from build123d import *

# Parameters (mm, degrees)
F0_W     = 261.6643384099
F0_H     = 143.3737166226
F1_DEPTH = 5
F2_R     = 19.4105187662
F3_DEPTH = 2
F6_R     = 6.5980928428
F7_DEPTH = 96.0488122602


# Not quite as in the source:
# - a feature of the source that left no trace in its solid (it failed there, or was rolled back) is left out


with BuildPart() as f1:
    # F0 (on Top) → F1 (new body)
    with BuildSketch(Plane.XY):
        with Locations((-11.2871490419, -11.1323576421)):
            Rectangle(F0_W, F0_H)
    extrude(amount=F1_DEPTH)

    # F2 (on face) → F3 (cut)
    with BuildSketch(Plane.XY.offset(5)):
        with Locations((-101.0480299592, -26.7270803452)):
            Circle(F2_R)
    extrude(amount=-F3_DEPTH, mode=Mode.SUBTRACT)


with BuildPart() as f7:
    # F6 (on line) → F7 (new body, through all)
    with BuildSketch(Plane(origin=(41.3091172937, 0, 32.6350144213), x_dir=(0, 1, 0), z_dir=(0.7846743667, 0, 0.6199081692))):
        with Locations((0, 4.5975914841)):
            Circle(F6_R)
    extrude(amount=-F7_DEPTH)


with BuildPart() as f1_1:
    add(f1.part)

    # F8: cut F7
    add(f7.part, mode=Mode.SUBTRACT)


solid = f1_1.part
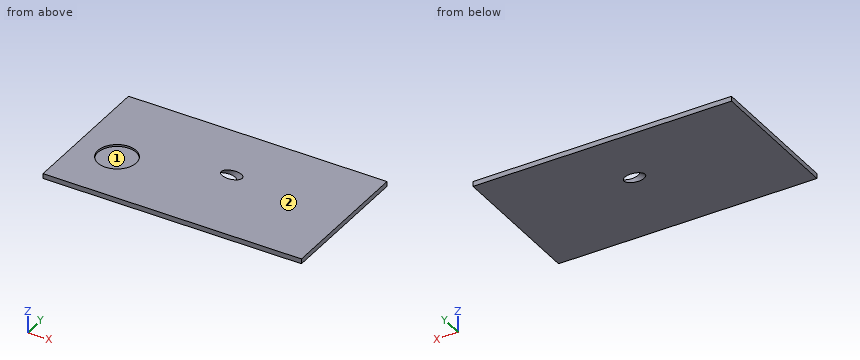
Verification items for the finished model (mm, model axes). Face numbers are marked on the shaded views. Give positions to 0.01 mm unless a question says otherwise; leave off trailing zeros. Loops run counter-clockwise (first coordinate to the right, second up) from the corner with the lowest first, then second, coordinate; pieces in that order, holes last. Notation, with made-up numbers: (-28, 20.25) - (-18, 20.25) arc R27 cw to (-18, 42.25) - close; hole circle Ø4 at (-27, -7). An arc over 180 degrees is marked (long way). Write item = value, one per line. Start each with the question number.
Q1. Cross-section at A-A, the plane y = 3. Enter the section's corners in (x, z).
Q2. Mould release check, pull along X, two halves, no side actions. Record for the marked faces 1 and 2: released by +X, released by -X, zero draft, split by the parting line, or undercut.
Q3. Thickness scan on line 1 (Y direction, x = -11, z = 1.1); line 2 (Y direction, x = -91, z = 3.65). Record the ranges inside material, lowest first.
Q4. Cross-section at B-B, the plane y = -32. Enter the section's corners in (x, z), and give its area (3 significant figures).
Q5. Cross-section at C-C, the plane z = 3.85. State how many separate pieces and enclosed holes the cut face has, and give its area (3 significant figures).
Answer key:
q1.outline = (-142.12, 0) - (-16.9, 0) - (-10.57, 5) - (-142.12, 5) - close; (2.06, 0) - (119.55, 0) - (119.55, 5) - (8.39, 5) - close
q2.face_1 = undercut
q2.face_2 = zero draft
q3.line_1 = -82.82 to -5.83, 5.83 to 60.55
q3.line_2 = -82.82 to -43.33, -10.12 to 60.55
q4.outline = (-142.12, 0) - (119.55, 0) - (119.55, 5) - (-82.37, 5) - (-82.37, 3) - (-119.73, 3) - (-119.73, 5) - (-142.12, 5) - close
q4.area = 1,230 mm^2
q5.separate_pieces = 1
q5.enclosed_holes = 2
q5.area = 36,100 mm^2
